Design review of the part shown in the three views and the two pictorial views. Dimensions are in mm from the part's minimum x, y and z. A direction names the side the tool comes from. Give positions to 0.01 mm unless a question says otherwise; leave off trailing zeros. Loops run counter-clockwise (first coordinate to the right, second up) from the corner with the lowest first, then second, coordinate; pieces in that order, holes last.
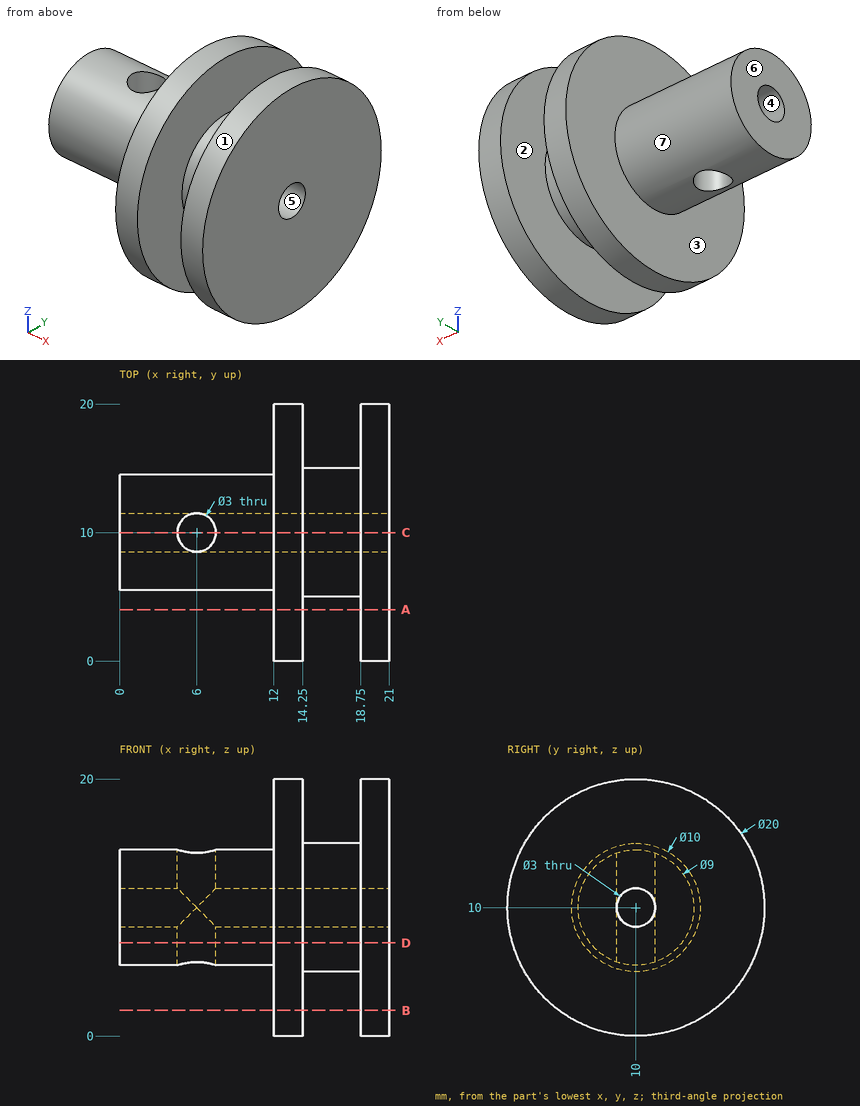
Q1. Consider section C-C on y = 10. Give the boundary of the cut face in (x, z).
Answers:
outline: (0, 5.5) - (4.5, 5.5) - (4.5, 8.5) - (0, 8.5) - close; (0, 11.5) - (4.5, 11.5) - (4.5, 14.5) - (0, 14.5) - close; (7.5, 5.5) - (12, 5.5) - (12, 0) - (14.25, 0) - (14.25, 5) - (18.75, 5) - (18.75, 0) - (21, 0) - (21, 8.5) - (7.5, 8.5) - close; (7.5, 11.5) - (21, 11.5) - (21, 20) - (18.75, 20) - (18.75, 15) - (14.25, 15) - (14.25, 20) - (12, 20) - (12, 14.5) - (7.5, 14.5) - close
Q2. For probe 1 along X at (y, z) = (10, 13.55); probe 2 along Y at (x, z) = (3.95, 10); probe 3 along X at (y, z) = (4.5, 18.25), list the stretches that pass through material, from the lowest coordinate up.
Answers:
probe 1: x = 0 to 4.5, 7.5 to 21
probe 2: y = 5.5 to 8.5, 11.5 to 14.5
probe 3: x = 12 to 14.25, 18.75 to 21
Q3. Consider section A-A on y = 4. Give the boundary of the cut face in (x, z), plus the area to 3 significant figures.
Answers:
outline: (12, 2) - (14.25, 2) - (14.25, 18) - (12, 18) - close; (18.75, 2) - (21, 2) - (21, 18) - (18.75, 18) - close
area: 72.0 mm2
Q4. For pin 1 Ø1 at (x, y) = (7, 6.5) entering from +Z; pin 2 Ø1 at (x, z) = (17, 7) entering from -Y; pin 3 Ø1.5 at (x, z) = (4, 6.5) entering from -Y; pin 4 Ø5 at (y, z) = (10, 10) entering from -X, all flat-tipped, find the tip position at first contact; note any pin that passes through.
Answers:
pin 1: stops at z = 13.35
pin 2: stops at y = 5.67
pin 3: stops at y = 6.44
pin 4: stops at x = 0
Q5. Mouldability with a two-part tool opening along Z and no side actions: class the marked faces 4, 5, 6 and 7 as +Z half, -Z half, draft (parallel to the pull), parting line (faces both ways), or undercut.
Answers:
face 4: undercut
face 5: undercut
face 6: draft
face 7: parting line
Q6. Consider section B-B on z = 2. Give the boundary of the cut face in (x, y), plus the area to 3 significant figures.
Answers:
outline: (12, 4) - (14.25, 4) - (14.25, 16) - (12, 16) - close; (18.75, 4) - (21, 4) - (21, 16) - (18.75, 16) - close
area: 54.0 mm2
Q7. Consider section D-D on z = 7.25. Give the boundary of the cut face in (x, y), plus the area to 3 significant figures.
Answers:
outline: (0, 6.44) - (12, 6.44) - (12, 0.39) - (14.25, 0.39) - (14.25, 5.82) - (18.75, 5.82) - (18.75, 0.39) - (21, 0.39) - (21, 19.61) - (18.75, 19.61) - (18.75, 14.18) - (14.25, 14.18) - (14.25, 19.61) - (12, 19.61) - (12, 13.56) - (0, 13.56) - close; hole circle Ø3 at (6, 10)
area: 203 mm2
Q8. Machinability: for the marked faces 1, 2 and 3, which of the approach directions +Z, -Z, +X, -X, +Y, -Y give a long, thin tool a straight path to every point of the face, cutting with its end or side? Answer none if there is none.
Answers:
face 1: +X, -X
face 2: none
face 3: -X
